from build123d import *

# Parameters (mm, degrees)
CROQUIS1_W              = 220
CROQUIS1_H              = 220
CROQUIS1_W_2            = 190
CROQUIS1_H_2            = 190
SALIENTE_EXTRUIR1_DEPTH = 10
REDONDEO2_R             = 4
CORTAR_EXTRUIR4_DEPTH   = 10
CORTAR_EXTRUIR5_DEPTH   = 10
CROQUIS6_W              = 214.832400875
CROQUIS6_H              = 220
CORTAR_EXTRUIR6_DEPTH   = 10
CROQUIS7_R              = 2.45
SALIENTE_EXTRUIR2_DEPTH = 5
CROQUIS11_W             = 15
CROQUIS11_H             = 15
CORTAR_EXTRUIR9_DEPTH   = 10
CROQUIS12_R             = 2.5
CORTAR_EXTRUIR10_DEPTH  = 6


with BuildPart() as part:
    # Croquis1 → Saliente-Extruir1 (new body)
    with BuildSketch(Plane.XY):
        with Locations((110, -110)):
            Rectangle(CROQUIS1_W, CROQUIS1_H)
        with Locations((110, -110)):
            Rectangle(CROQUIS1_W_2, CROQUIS1_H_2, mode=Mode.SUBTRACT)
        Polygon((212.5, -13.273502692), (217.5, -10.386751346), (217.5, -4.613248654), (212.5, -1.726497308), (207.5, -4.613248654), (207.5, -10.386751346), align=None, mode=Mode.SUBTRACT)
        Polygon((7.5, -13.273502692), (12.5, -10.386751346), (12.5, -4.613248654), (7.5, -1.726497308), (2.5, -4.613248654), (2.5, -10.386751346), align=None, mode=Mode.SUBTRACT)
        Polygon((212.5, -218.273502692), (217.5, -215.386751346), (217.5, -209.613248654), (212.5, -206.726497308), (207.5, -209.613248654), (207.5, -215.386751346), align=None, mode=Mode.SUBTRACT)
        Polygon((7.5, -218.273502692), (12.5, -215.386751346), (12.5, -209.613248654), (7.5, -206.726497308), (2.5, -209.613248654), (2.5, -215.386751346), align=None, mode=Mode.SUBTRACT)
    extrude(amount=SALIENTE_EXTRUIR1_DEPTH)

    # Redondeo2
    redondeo2_edges = [part.edges().sort_by_distance(p)[0] for p in [
        (0, 0, 5),
        (220, 0, 5),
        (220, -220, 5),
        (0, -220, 5),
    ]]
    fillet(redondeo2_edges, radius=REDONDEO2_R)

    # Croquis4 → Cortar-Extruir4 (cut)
    with BuildSketch(Plane.XY.offset(10)):
        with BuildLine():
            Line((42.5, -4.5), (177.5, -4.5))
            ThreePointArc((177.5, -4.5), (180.5, -7.5), (177.5, -10.5))
            Line((177.5, -10.5), (42.5, -10.5))
            ThreePointArc((42.5, -10.5), (39.5, -7.5), (42.5, -4.5))
        make_face()
        with BuildLine():
            Line((42.5, -215.5), (177.5, -215.5))
            ThreePointArc((177.5, -215.5), (180.5, -212.5), (177.5, -209.5))
            Line((177.5, -209.5), (42.5, -209.5))
            ThreePointArc((42.5, -209.5), (39.5, -212.5), (42.5, -215.5))
        make_face()
    extrude(amount=-CORTAR_EXTRUIR4_DEPTH, mode=Mode.SUBTRACT)

    # Croquis5 → Cortar-Extruir5 (cut)
    with BuildSketch(Plane.XY.offset(10)):
        with BuildLine():
            Line((10.5, -42.5), (10.5, -177.5))
            ThreePointArc((10.5, -177.5), (7.5, -180.5), (4.5, -177.5))
            Line((4.5, -177.5), (4.5, -42.5))
            ThreePointArc((4.5, -42.5), (7.5, -39.5), (10.5, -42.5))
        make_face()
        with BuildLine():
            Line((209.5, -42.5), (209.5, -177.5))
            ThreePointArc((209.5, -177.5), (212.5, -180.5), (215.5, -177.5))
            Line((215.5, -177.5), (215.5, -42.5))
            ThreePointArc((215.5, -42.5), (212.5, -39.5), (209.5, -42.5))
        make_face()
    extrude(amount=-CORTAR_EXTRUIR5_DEPTH, mode=Mode.SUBTRACT)

    # Croquis6 → Cortar-Extruir6 (cut)
    with BuildSketch(Plane.XY.offset(10)):
        with Locations((122.416200438, -110)):
            Rectangle(CROQUIS6_W, CROQUIS6_H)
    extrude(amount=-CORTAR_EXTRUIR6_DEPTH, mode=Mode.SUBTRACT)

    # Croquis7 → Saliente-Extruir2 (add)
    with BuildSketch(Plane(origin=(15, 0, 0), x_dir=(0, 0, -1), z_dir=(1, 0, 0))):
        with Locations((-5, -7.5)):
            Circle(CROQUIS7_R)
    extrude(amount=SALIENTE_EXTRUIR2_DEPTH)

    # Croquis11 → Cortar-Extruir9 (cut)
    with BuildSketch(Plane.XY.offset(10)):
        with Locations((7.5, -212.5)):
            Rectangle(CROQUIS11_W, CROQUIS11_H)
    extrude(amount=-CORTAR_EXTRUIR9_DEPTH, mode=Mode.SUBTRACT)

    # Croquis12 → Cortar-Extruir10 (cut)
    with BuildSketch(Plane.XZ.offset(205)):
        with Locations((7.5, 5)):
            Circle(CROQUIS12_R)
    extrude(amount=-CORTAR_EXTRUIR10_DEPTH, mode=Mode.SUBTRACT)


solid = part.part
Here's how the part is built. I have some questions about the finished solid (model axes, mm). A direction names the side the tool comes from. Round coordinates to 2 decimals unless told otherwise and drop trailing zeros. Loops run counter-clockwise (first coordinate to the right, second up) from the corner with the lowest first, then second, coordinate; pieces in that order, holes last. Notation, with made-up numbers: (-29.75, -27) -> (0.25, -27) arc R23 ccw to (0.25, 3) -> close; hole circle Ø7 at (49, 24). An arc over 180 degrees is marked (long way). Write each question's results on one line, items separated by ' | '.
(1) If I drill on L1, parallel to Y at x = 5.25, z = 2.5; L2, parallel to Z at x = 7.5, y = -203.3; L3, parallel to Y at x = 5.5, z = 4.25, over which ranges is the centre line in solid material (lowest first)?
Worked answers:
L1: -205 to -179.48, -40.52 to -11.97, -3.03 to 0 | L2: 0 to 2.5, 7.5 to 10 | L3: -199 to -179.74, -40.26 to -12.12, -2.88 to 0
(2) If we section it at C-C, the plane y = -7.5: List the corners of the cut face in (x, z) for me, then the cut area to 3 significant figures.
Worked answers:
outline: (0, 0) -> (2.5, 0) -> (2.5, 10) -> (0, 10) -> close; (12.5, 0) -> (15, 0) -> (15, 2.55) -> (20, 2.55) -> (20, 7.45) -> (15, 7.45) -> (15, 10) -> (12.5, 10) -> close | area: 74.5 mm2
(3) For faces 1 (the face through (7.6, -180.5, 5.1)), 2 (the face through (1.141, -1.203, 5.07)), 3 (the face through (9.885, -202.042, 5.751)), 4 (the face through (17.465, -9.674, 3.869)), which set-ups out of +Z, -Z, +X, -X, +Y, -Y let a thin tool reach every point of the face, with its end or its side?
Worked answers:
face 1: +Z, -Z | face 2: +Z, -Z, -X, +Y | face 3: -Y | face 4: +X
(4) If we section it at B-B, the plane z = 5: List the corners of the cut face in (x, y) for me, then the cut area to 3 significant figures.
Worked answers:
outline: (0, -205) -> (5, -205) -> (5, -199) -> (10, -199) -> (10, -205) -> (15, -205) -> (15, -9.95) -> (20, -9.95) -> (20, -5.05) -> (15, -5.05) -> (15, 0) -> (4, 0) arc R4 ccw to (0, -4) -> close; hole (2.5, -10.39) -> (7.5, -13.27) -> (12.5, -10.39) -> (12.5, -4.61) -> (7.5, -1.73) -> (2.5, -4.61) -> close; hole (4.5, -177.5) arc R3 ccw to (10.5, -177.5) -> (10.5, -42.5) arc R3 ccw to (4.5, -42.5) -> close | area: 2,140 mm2
(5) For P1, Ø3, axis at y = -125, z = 3, coming from the +X side; P2, Ø1.5, axis at x = 7.5, z = 4, coming from the -Y side, each with a flat end and sliding along its axis, tell me the tip position at first contact or that it passes through.
Worked answers:
P1: x = 15 | P2: y = -199
(6) We'd pull the mould along Z, two halves only. Please class faces 5 (the face through (4, -101, 0)), 6 (the face through (7, -199, 5)), 7 (the face through (5.035, -3.15, 4.93)): released by +Z, released by -Z, zero draft, split by the parting line, or undercut.
Worked answers:
face 5: released by -Z | face 6: undercut | face 7: zero draft
(7) If we section it at A-A, the plane y = -73: List the corners of the cut face in (x, z) for me, then the cut area to 3 significant figures.
Worked answers:
outline: (0, 0) -> (4.5, 0) -> (4.5, 10) -> (0, 10) -> close; (10.5, 0) -> (15, 0) -> (15, 10) -> (10.5, 10) -> close | area: 90.0 mm2
